Autodesk Inventor part; units mm, degrees
ref_plane "YZ Plane" through (0, 0, 0) normal (1, 0, 0) x (0, 1, 0)
ref_plane "XZ Plane" through (0, 0, 0) normal (0, 1, 0) x (-1, 0, 0)
ref_plane "XY Plane" through (0, 0, 0) normal (0, 0, 1) x (1, 0, 0)
sketch "Sketch1" plane through (0, 0, 0) normal (0, 0, 1) x (1, 0, 0)
  line L0 (12.5, 17.5) -> (-12.5, 17.5)
  line L1 (-12.5, 17.5) -> (-12.5, -17.5)
  line L2 (-12.5, -17.5) -> (12.5, -17.5)
  line L3 (12.5, -17.5) -> (12.5, 17.5)
  point P0 (0, 0)
  point P1 (12.5, 0)
  dimension "d0" = 25
  dimension "d1" = 35
  dimension "d16" = 12.5
extrude "Extrusion1" add sketch "Sketch1" along normal blind 12
sketch "Sketch2" plane through (0, 0, 12) normal (0, 0, 1) x (1, 0, 0)
  circle A0 centre (0, 0) radius 3.05
  dimension "d4" = 6.1
extrude "Extrusion2" cut sketch "Sketch2" against normal up to next
sketch "Sketch4" plane through (0, 0, 12) normal (0, 0, 1) x (1, 0, 0)
  circle A0 centre (0, 0) radius 3.05
  arc A1 (-7, -3.0859) -> (-5.7899, 5) centre (0, 0) ccw
  line L0 (-5.7899, 5) -> (-11, 5)
  line L1 (-11, 5) -> (-11, -17.5)
  line L2 (-12.5, -17.5) -> (12.5, -17.5)
  line L3 (-7, -3.0859) -> (-7, -17.5)
  circle A2 centre (0, 0) radius 3.05
  line L4 (12.5, 17.5) -> (-12.5, 17.5)
  line L5 (-12.5, 17.5) -> (-12.5, -17.5)
  line L6 (-12.5, -17.5) -> (12.5, -17.5)
  line L7 (12.5, -17.5) -> (12.5, 17.5)
  dimension "d9" = 15.3
  dimension "d10" = 11
  dimension "d11" = 7
  dimension "d12" = 5
extrude "Extrusion3" add sketch "Sketch4" along normal blind 15 contours A1 L0 L1 L2 L5 L4 L7 L3
fillet "Fillet1" radius 2 3 edges at (-7, -3.0859, 19.5) (-5.7899, 5, 19.5) (-11, 5, 19.5)
sketch "Sketch5" plane through (0, 0, 27) normal (0, 0, 1) x (1, 0, 0)
  point P0 (0, 0)
  point P1 (-8, 12)
  point P2 (7, -12)
  dimension "d17" = 7
  dimension "d18" = 12
  dimension "d19" = 12
  dimension "d20" = 8
hole "Hole1" at (-8, 12, 27) at (7, -12, 27) direction (0, 0, -1) diameter 4.2 depth 8 tip angle 118 countersink diameter 6 countersink angle 90
chamfer "Chamfer1" distance 1 angle 45 6 edges at (7.606, 0.819, 27) (-5.9817, -6.5111, 27) (-7, -12.8768, 27) (-5.9014, 5.1424, 27) (-7.8212, 5, 27) (-11, -7.25, 27)
properties part number "Base" material "ABS Plastic"
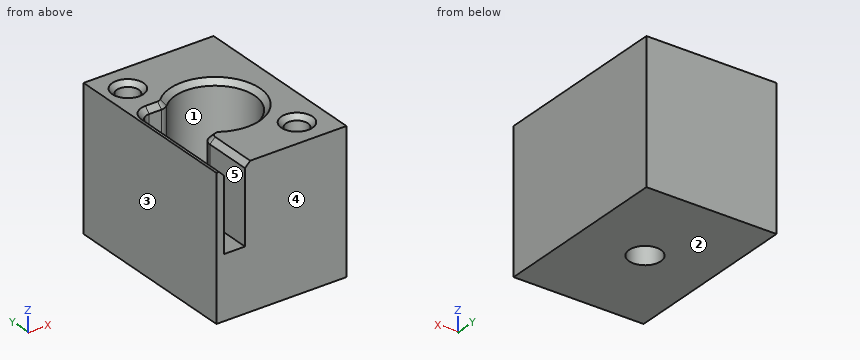
Check sheet for the modelled part. Datum: model origin and axes. Units: mm. Face numbers are marked on the shaded views. A direction names the side the tool comes from. Round coordinates to 2 decimals unless told otherwise and drop trailing zeros. Order: outer loops, then holes, each group sorted by start corner. A loop starts at its lowest first (then second) coordinate and runs counter-clockwise, first axis right, second up. Notation, with made-up numbers: (63, 10.25) -> (90, 10.25) arc R28 ccw to (90, 37.25) -> close; hole circle Ø11 at (36.5, -18.75). An arc over 180 degrees is marked (long way). One line per item, written item: value. Start each with the question number.
Q1. Cross-section at A-A (z = 19.75). Record the boundary of the cut face in (x, y).
Q2. Mould release check, pull along X, two halves, no side actions. Record for the marked faces 3, 4 and 5: pulls with the +X half, pulls with the -X half, needs draft (parallel to the pull), parting line crosses it, or undercut.
Q3. Set-up check for the marked faces 1 and 2: record each of +Z, -Z, +X, -X, +Y, -Y from which the full face is reachable in a straight line by a thin tool's end or side.
Q4. Thickness scan on line 1 (X direction, y = -16, z = 24.5); line 2 (X direction, y = -12, z = 23.75); line 3 (X direction, y = 12, z = 23.25). Record the ranges inside material, lowest first.
Q5. Gauge pin test, flat ends, axial feed: pin 1 Ø2.5 at (x, y) = (7, -12) entering from +Z; pin 2 Ø1.2 at (x, z) = (-8.5, 21.5) entering from -Y; pin 3 Ø5.5 at (x, y) = (0, 0) entering from -Z (1 decimal). Record the tip position at first contact, or that the pin passes through.
Completed:
1. outline: (-12.5, -17.5) -> (-11, -17.5) -> (-11, 3) arc R2 cw to (-9, 5) -> (-6.64, 5) arc R2 ccw to (-5.27, 5.55) arc R7.65 cw (long way) to (-3.96, -6.54) arc R2 ccw to (-7, -8.25) -> (-7, -17.5) -> (12.5, -17.5) -> (12.5, 17.5) -> (-12.5, 17.5) -> close; hole circle Ø4.2 at (-8, 12); hole circle Ø4.2 at (7, -12)
2. face 3: pulls with the -X half
2. face 4: needs draft
2. face 5: undercut
3. face 1: +Z
3. face 2: -Z, +X, -X, +Y, -Y
4. line 1: x = -12.5 to -11, -7 to 12.5
4. line 2: x = -12.5 to -11, -7 to 4.9, 9.1 to 12.5
4. line 3: x = -12.5 to -10.1, -5.9 to 12.5
5. pin 1: stops at z = 18.49
5. pin 2: stops at y = 5
5. pin 3: passes through
